Job drawing, mm, ordinate dimensions from the low corner. One solid piece. Give positions to 0.01 mm unless a question says otherwise; leave off trailing zeros. Order: outer loops, then holes, each group sorted by start corner. A loop starts at its lowest first (then second) coordinate and runs counter-clockwise, first axis right, second up. Notation, with made-up numbers: M 23.25,32 L 36.25,32 A32 ccw 36.25,68 Z; hole C -6,-18 d2. An arc over 180 degrees is marked long. One line per item, written item: value. Start each with the question number.
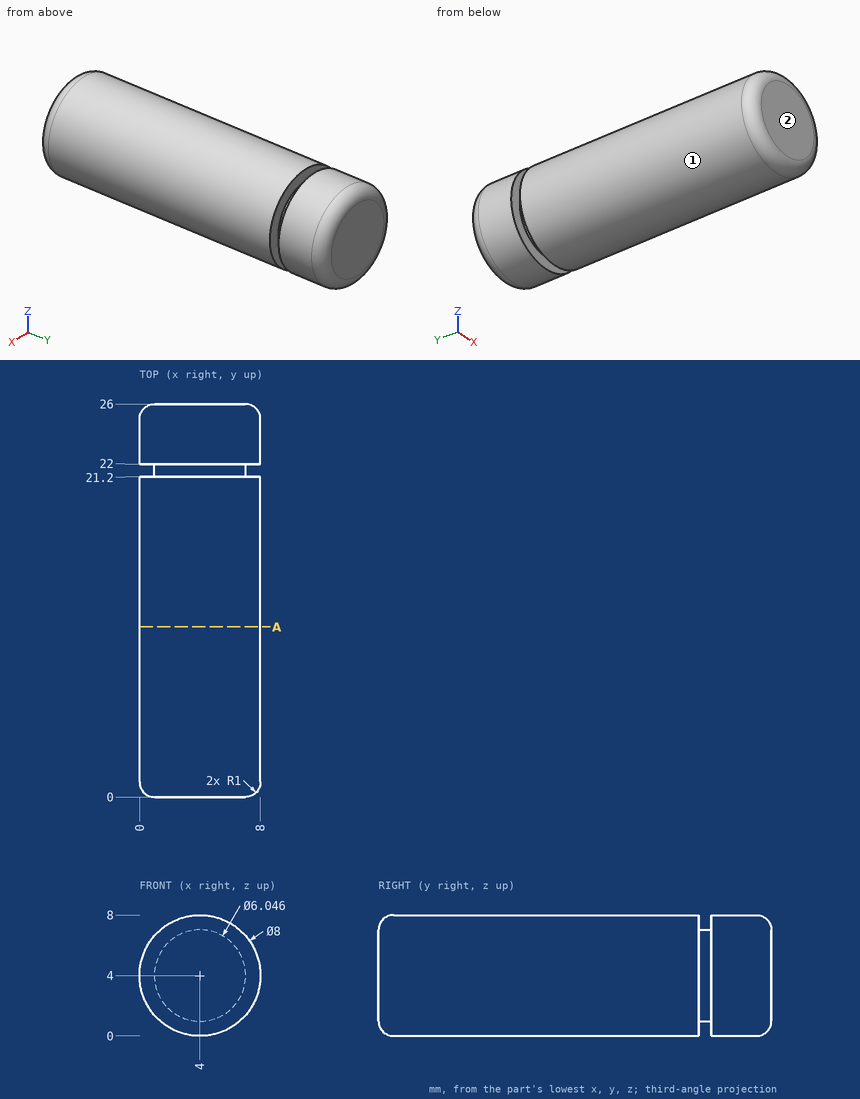
1) Slice it at A-A (y = 11.25). List the corners of the cut face in (x, z).
2) Drill centre lines: line 1 (Y direction, x = 7.25, z = 2); line 2 (Y direction, x = 6.75, z = 2.5); line 3 (Z direction, x = 1.75, y = 23.25). Where is each one in solid material? Low to high.
3) Drop a flat-ended pin along its axis: P1, Ø3, axis at x = 7, y = 21, coming from the -Z side. Give the stop position or say it passes through.
4) Pull direction Z, two halves, no side cores. Call the marked faces 1 and 2: pulls with the +Z half, pulls with the -Z half, needs draft (parallel to the pull), parting line crosses it, or undercut.
Results list:
1. outline: C 4,4 d8
2. line 1: y = 0.42 to 21.2, 22 to 25.58
2. line 2: y = 0.01 to 21.2, 22 to 25.99
2. line 3: z = 0.69 to 7.31
3. P1: stops at z = 0.29
4. face 1: parting line crosses it
4. face 2: needs draft
